Autodesk Inventor part; units mm, degrees
ref_plane "YZ Plane" through (0, 0, 0) normal (1, 0, 0) x (0, 1, 0)
ref_plane "XZ Plane" through (0, 0, 0) normal (0, 1, 0) x (-1, 0, 0)
ref_plane "XY Plane" through (0, 0, 0) normal (0, 0, 1) x (1, 0, 0)
sketch "Sketch1" plane through (0, 0, 0) normal (0, 0, 1) x (1, 0, 0)
  circle A0 centre (0, 0) radius 15
  circle A1 centre (0, 0) radius 5
  circle A2 centre (-12.5, 0) radius 1.4
  circle A3 centre (0, -12.5) radius 1.4
  circle A4 centre (12.5, 0) radius 1.4
  circle A5 centre (0, 12.5) radius 1.4
  line L0 (0, -15) -> (1.0439, -14.9636)
  line L1 (100, 15) -> (70, 15)
  line L2 (70, -12.5614) -> (70, -15)
  line L3 (70, -15) -> (100, -15)
  line L4 (100, -15) -> (100, 15)
  line L5 (100, 15) -> (70, -15) construction
  line L6 (70, 15) -> (100, -15) construction
  circle A6 centre (100, 0) radius 12.2
  line L7 (0, 15) -> (100, 15)
  line L8 (0, -15) -> (100, -15)
  point P0 (85, 0)
  point P1 (100, -12.2)
  point P2 (100, 12.2)
  dimension "d0" = 30
  dimension "d1" = 10
  dimension "d2" = 2.8
  dimension "d3" = 12.5
  dimension "d6" = 360
  dimension "d9" = 30
  dimension "d10" = 30
  dimension "d11" = 24.4
  dimension "d12" = 100
extrude "Extrusion1" add sketch "Sketch1" along normal blind 5 contours A0 L0 | A0 L7 L1 L4 A6 L3 L8 picked at (9.3778, -4.158)
sketch "Sketch2" plane through (0, 15, 0) normal (0, 1, 0) x (1, 0, 0)
  point P0 (0, 0)
sketch "Sketch3" plane through (0, 0, 5) normal (0, 0, 1) x (1, 0, 0)
  line L0 (100, 15) -> (0, 15)
  line L1 (0, -15) -> (100, -15)
  line L2 (81.3075, 15) -> (100, 15)
  line L3 (100, 15) -> (100, -15)
  line L4 (100, -15) -> (81.3075, -15)
  line L5 (81.3075, -15) -> (81.3075, 15)
  circle A0 centre (100, 0) radius 12.2
  point P0 (0, 0)
  point P1 (100, -12.2)
  point P2 (100, 12.2)
  dimension "d15" = 24.4
extrude "Extrusion2" add sketch "Sketch3" along normal blind 10 contours L3 A0 L1 L5 L0
sketch "Sketch4" plane through (0, 15, 0) normal (0, 1, 0) x (1, 0, 0)
  line L0 (100, 0) -> (100, -15)
  line L1 (100, 0) -> (87.8, 0)
  line L2 (100, -15) -> (90, -15)
  line L3 (90, -15) -> (90, 0)
  line L4 (90, 0) -> (100, 0)
  line L5 (100, 0) -> (100, -15)
  point P0 (0, 0)
  dimension "d18" = 10
extrude "Extrusion3" add sketch "Sketch4" along normal blind 10
sketch "Sketch5" plane through (0, -15, 0) normal (0, -1, 0) x (1, 0, 0)
  line L0 (100, 0) -> (100, 15)
  line L1 (100, 15) -> (90, 15)
  line L2 (90, 15) -> (90, 0)
  line L3 (90, 0) -> (100, 0)
  line L4 (100, 0) -> (100, 15)
  point P0 (0, 0)
  dimension "d21" = 10
  dimension "d22" = 15
extrude "Extrusion4" add sketch "Sketch5" along normal blind 10
sketch "Sketch6" plane through (100, -12.2, 15) normal (1, 0, 0) x (0, 0, -1)
  circle A0 centre (7.5, -7.8) radius 1.4
  line L0 (15, -12.8) -> (0, -12.8)
  line L1 (0, 0) -> (0, -12.8)
  line L2 (15, 12.2) -> (0, 12.2)
  line L3 (0, 0) -> (0, 24.4)
  circle A1 centre (7.5, 32.2) radius 1.4
  dimension "d25" = 2.8
  dimension "d26" = 5
  dimension "d27" = 7.5
extrude "Extrusion5" cut sketch "Sketch6" against normal through all
fillet "Fillet1" radius 2 2 edges at (95, -25, 0) (95, -25, 15)
fillet "Fillet2" radius 2 2 edges at (95, 25, 0) (95, 25, 15)
sketch "Sketch7" plane through (0, 0, 0) normal (0, 0, -1) x (-1, 0, 0)
  line L0 (-81.3075, 15) -> (-81.3075, -15)
  line L1 (-17.3755, -15) -> (-81.3075, -15)
  line L2 (-81.3075, -15) -> (-81.3075, 15)
  line L3 (-81.3075, 15) -> (-17.3755, 15)
  line L4 (-17.3755, 15) -> (-17.3755, -15)
  line L5 (-25.565, -7.4736) -> (-75.565, -7.4736) construction
  line L6 (-25.565, -4.9736) -> (-75.565, -4.9736)
  line L7 (-75.565, -9.9736) -> (-25.565, -9.9736)
  arc A0 (-25.565, -9.9736) -> (-25.565, -4.9736) centre (-25.565, -7.4736) ccw
  arc A1 (-75.565, -4.9736) -> (-75.565, -9.9736) centre (-75.565, -7.4736) ccw
  line L8 (-25.565, 6.3477) -> (-75.565, 6.3477) construction
  line L9 (-25.565, 3.8477) -> (-75.565, 3.8477)
  line L10 (-75.565, 8.8477) -> (-25.565, 8.8477)
  arc A2 (-25.565, 3.8477) -> (-25.565, 8.8477) centre (-25.565, 6.3477) ccw
  arc A3 (-75.565, 8.8477) -> (-75.565, 3.8477) centre (-75.565, 6.3477) ccw
  point P0 (0, 0)
  point P1 (-50.565, -7.4736)
  point P2 (-50.565, 6.3477)
  dimension "d32" = 30
  dimension "d33" = 5
  dimension "d34" = 50
  dimension "d35" = 50
  dimension "d36" = 2.5
extrude "Extrusion6" cut sketch "Sketch7" against normal through all contours A0 L7 A1 L6 | L9 A3 L10 A2
fillet "Fillet3" radius 2 2 edges at (85.6537, 15, 15) (85.6537, -15, 15)
sketch "Sketch8" plane through (90, 15, 0) normal (-1, 0, 0) x (0, 0, 1)
  point P0 (0, -15)
properties part number "link1"
Source: CAD feature listing. Evaluate the final solid. Frame: model axes, mm. A direction names the side the tool comes from. Round coordinates to 2 decimals unless told otherwise and drop trailing zeros. Loops run counter-clockwise (first coordinate to the right, second up) from the corner with the lowest first, then second, coordinate; pieces in that order, holes last. Notation, with made-up numbers: (-3.5, 9.25) - (3.5, 9.25) arc R31 cw to (3.5, 48.25) - close; hole circle Ø2 at (77.5, -29.75). An arc over 180 degrees is marked (long way). Use CSV: the item, a comma, the result in double quotes.
Q1. Mould query, pull axis Y, two halves, no side actions, for faces 3 (the cylindrical face through (85.59, 14.4, 14.43)), 4 (the flat face through (100, 17, 7)), 5 (the cylindrical face through (95.07, -24.43, 0.6)), 6 (the cylindrical face through (0.75, 11.32, 2.46)). Classes: pulls with the +Y half, pulls with the -Y half, needs draft (parallel to the pull), parting line crosses it, or undercut.
Reported:
face 3,"pulls with the +Y half"
face 4,"needs draft"
face 5,"pulls with the -Y half"
face 6,"undercut"
Q2. Reachability of faces 1 (the cylindrical face through (23.066, 6.293, 2.465)), 2 (the cylindrical face through (-15, 0, 2)) from +Z, -Z, +X, -X, +Y, -Y: full face, straight path, thin tool, end or side. Return the list, or none.
Reported:
face 1,"+Z, -Z"
face 2,"+Z, -Z, -X"
Q3. Section query D-D, the plane y = -20. Output: boundary loops of the cut face in (x, z), then the cut area to 3 significant figures.
Reported:
outline,"(90, 0) - (100, 0) - (100, 6.1) - (90, 6.1) - close; (90, 8.9) - (100, 8.9) - (100, 15) - (90, 15) - close"
area,"122 mm^2"
Q4. Pin query (flat end, axial travel): pin 1 Ø5.5 at (x, z) = (54.5, 2) entering from -Y; pin 2 Ø6 at (y, z) = (-16.5, 8) entering from -X; pin 3 Ø8 at (y, z) = (-1.5, 10.5) entering from +X; pin 4 Ø6 at (x, y) = (57, -19.5) entering from +Z. Return the tip coordinate at first contact, or that it passes through.
Reported:
pin 1,"y = -15"
pin 2,"x = 81.31"
pin 3,"x = 89.11"
pin 4,"through"
Q5. Section query C-C, the plane z = 7.5. Output: boundary loops of the cut face in (x, y), then the cut area to 3 significant figures.
Reported:
outline,"(81.31, -15) - (90, -15) - (90, -18.6) - (100, -18.6) - (100, -12.2) arc R12.2 cw to (100, 12.2) - (100, 18.6) - (90, 18.6) - (90, 15) - (81.31, 15) - close; (90, -25) - (100, -25) - (100, -21.4) - (90, -21.4) - close; (90, 21.4) - (100, 21.4) - (100, 25) - (90, 25) - close"
area,"471 mm^2"
Q6. Section query A-A, the plane y = 0. Output: boundary loops of the cut face in (x, z), then the cut area to 3 significant figures.
Reported:
outline,"(-15, 0) - (-13.9, 0) - (-13.9, 5) - (-15, 5) - close; (-11.1, 0) - (-5, 0) - (-5, 5) - (-11.1, 5) - close; (5, 0) - (11.1, 0) - (11.1, 5) - (5, 5) - close; (13.9, 0) - (87.8, 0) - (87.8, 15) - (81.31, 15) - (81.31, 5) - (13.9, 5) - close"
area,"501 mm^2"
Q7. Section query B-B, the plane x = 33.5. Output: boundary loops of the cut face in (y, z).
Reported:
outline,"(-15, 0) - (-9.97, 0) - (-9.97, 5) - (-15, 5) - close; (-4.97, 0) - (3.85, 0) - (3.85, 5) - (-4.97, 5) - close; (8.85, 0) - (15, 0) - (15, 5) - (8.85, 5) - close"
Q8. Ray query, line 1 along Y through (x, z) = (58.5, 3.75); line 2 along Y through (x, z) = (91.5, 6.75); line 3 along Z through (x, y) = (-1, 6). Return the intervals inside material, ascending.
Reported:
line 1,"-15 to -9.97, -4.97 to 3.85, 8.85 to 15"
line 2,"-25 to -21.18, -18.82 to -8.75, 8.75 to 18.82, 21.18 to 25"
line 3,"0 to 5"
